from build123d import *

# Parameters (mm, degrees)
F0_R     = 17.5
F0_R_2   = 10.25
F1_DEPTH = 57.5
F2_R     = 2.4
F3_DEPTH = 25
F4_SIZE  = 1
F5_SIZE  = 1


with BuildPart() as f1:
    # F0 (on Top) → F1 (new body, symmetric)
    with BuildSketch(Plane.XY):
        Circle(F0_R)
        Circle(F0_R_2, mode=Mode.SUBTRACT)
    extrude(amount=F1_DEPTH, both=True)

    # F2 (on Front) → F3 (cut)
    with BuildSketch(Plane.XZ):
        Circle(F2_R)
    extrude(amount=F3_DEPTH, mode=Mode.SUBTRACT)

    # F4
    f4_edges = [f1.edges().sort_by_distance(p)[0] for p in [
        (-10.25, 0, 57.5),
    ]]
    chamfer(f4_edges, length=F4_SIZE)

    # F5
    f5_edges = [f1.edges().sort_by_distance(p)[0] for p in [
        (-10.25, 0, -57.5),
    ]]
    chamfer(f5_edges, length=F5_SIZE)


solid = f1.part
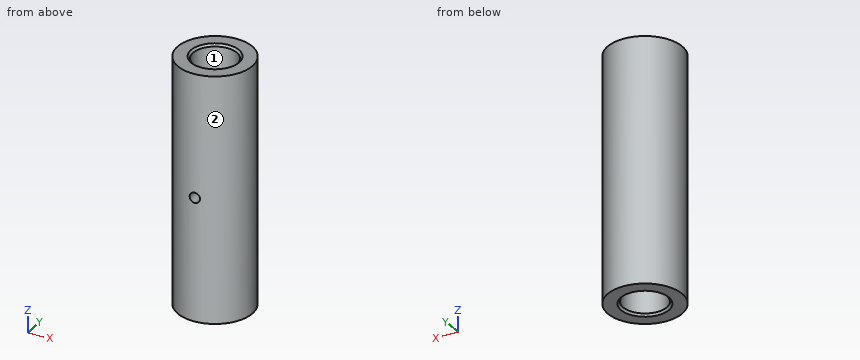
Design review of the part built by this model. Coordinates are the model's own, in mm. Face numbers are marked on the shaded views. Give positions to 0.01 mm unless a question says otherwise; leave off trailing zeros. Loops run counter-clockwise (first coordinate to the right, second up) from the corner with the lowest first, then second, coordinate; pieces in that order, holes last. Notation, with made-up numbers: (21.5, 8.5) - (57.5, 8.5) arc R20 ccw to (57.5, 24.5) - close; hole circle Ø4 at (7, 10.5). An arc over 180 degrees is marked (long way). Write item = value, one per line.
1) To check wall thickness, follow line 1 (Y direction, x = 0, z = 2.5); line 2 (Z direction, x = 0, y = -13); line 3 (Y direction, x = 6, z = 33). State the ranges of each line that lie inside material, in increasing order.
Result sheet:
line_1 = -17.5 to -10.25, 10.25 to 17.5
line_2 = -57.5 to -2.4, 2.4 to 57.5
line_3 = -16.44 to -8.31, 8.31 to 16.44
2) Take a section at B-B on y = 0. State the section outline as (x, z) points, and give its area (3 significant figures).
Result sheet:
outline = (-17.5, -57.5) - (-11.25, -57.5) - (-10.25, -56.5) - (-10.25, 56.5) - (-11.25, 57.5) - (-17.5, 57.5) - close; (10.25, -56.5) - (11.25, -57.5) - (17.5, -57.5) - (17.5, 57.5) - (11.25, 57.5) - (10.25, 56.5) - close
area = 1,670 mm2
3) Take a section at C-C on z = 38.5. State the section outline as (x, y) points, and give its area (3 significant figures).
Result sheet:
outline = circle Ø35 at (0, 0); hole circle Ø20.5 at (0, 0)
area = 632 mm2
4) Take a section at D-D on y = -15. State the section outline as (x, z) points, and give its area (3 significant figures).
Result sheet:
outline = (-9.01, -57.5) - (9.01, -57.5) - (9.01, 57.5) - (-9.01, 57.5) - close; hole circle Ø4.8 at (0, 0)
area = 2,060 mm2
5) Clearance check with flat-ended pins moving along their axes: pin 1 Ø1 at (y, z) = (3, -31) entering from -X; pin 2 Ø12 at (y, z) = (-7.5, 9.5) entering from -X; pin 3 Ø4 at (y, z) = (-13, 34) entering from +X. State where each tip first meets the part, or that it passes through.
Result sheet:
pin_1 = -17.32
pin_2 = -17.44
pin_3 = 13.61
6) Draft analysis for pull direction Y (two halves, no side actions). For the marked faces 1 and 2, state which applies: +Y half, -Y half, draft (parallel to the pull), parting line (faces both ways), or undercut.
Result sheet:
face_1 = undercut
face_2 = parting line
7) Take a section at A-A on x = 0. State the section outline as (y, z) points.
Result sheet:
outline = (-17.5, -57.5) - (-11.25, -57.5) - (-10.25, -56.5) - (-10.25, -2.4) - (-17.5, -2.4) - close; (-17.5, 2.4) - (-10.25, 2.4) - (-10.25, 56.5) - (-11.25, 57.5) - (-17.5, 57.5) - close; (10.25, -56.5) - (11.25, -57.5) - (17.5, -57.5) - (17.5, 57.5) - (11.25, 57.5) - (10.25, 56.5) - close
